Source: CAD feature listing. Evaluate the final solid. Frame: model axes, mm. Round coordinates to 2 decimals unless told otherwise and drop trailing zeros. Loops run counter-clockwise (first coordinate to the right, second up) from the corner with the lowest first, then second, coordinate; pieces in that order, holes last.
Item 1: Ray query, L1, parallel to Z at x = 5.45, y = 10; L2, parallel to Y at x = 4, z = 4; L3, parallel to Y at x = 1.8, z = -2. Return the intervals inside material, ascending.
Item 2: Section query B-B on z = 5. Return loops of the section in (x, y), then the cut area to 3 significant figures.
Item 3: Section query A-A on y = 10. Return loops of the section in (x, z), then the cut area to 3 significant figures.
Item 4: Section query D-D on y = 12.25. Return loops of the section in (x, z).
Item 5: Pull-direction query (Y, two-part tool) for faces 1 (the flat face through (3, 0, 12)), 2 (the cylindrical face through (2.96, 0.21, -0.43)), 3 (the flat face through (3, 0.2, 13)); classes: released by +Y, released by -Y, zero draft, split by the parting line, or undercut.
Item 6: Section query C-C on x = 5.5. Return loops of the section in (y, z).
Autodesk Inventor part; units mm, degrees
ref_plane "YZ Plane" through (0, 0, 0) normal (1, 0, 0) x (0, 1, 0)
ref_plane "XZ Plane" through (0, 0, 0) normal (0, 1, 0) x (-1, 0, 0)
ref_plane "XY Plane" through (0, 0, 0) normal (0, 0, 1) x (1, 0, 0)
sketch "Sketch1" plane through (0, 0, 0) normal (0, 0, 1) x (1, 0, 0)
  line L0 (0, 0) -> (6, 0)
  line L1 (6, 0) -> (6, 0.2)
  line L2 (6, 0.2) -> (0, 0.2)
  line L3 (0, 0.2) -> (0, 0)
  dimension "d0" = 0.2
  dimension "d1" = 6
extrude "Extrusion1" add sketch "Sketch1" along normal blind 10
sketch "Sketch2" plane through (0, 0, 0) normal (1, 0, 0) x (0, 1, 0)
  line L0 (0, 0) -> (0.2, 0)
  line L1 (0, 0) -> (10, 0)
  circle A0 centre (10, 0) radius 10
  circle A1 centre (10, 0) radius 9.8
  dimension "d4" = 10
extrude "Extrusion2" add sketch "Sketch2" along normal up to surface (6 mm away)
sketch "Sketch3" plane through (0, 0, 10) normal (0, 0, 1) x (1, 0, 0)
  line L0 (0, 0) -> (0, 0.2)
  line L1 (6, 0) -> (0, 0)
  line L2 (6, 0.2) -> (6, 0)
  line L3 (0, 0.2) -> (6, 0.2)
extrude "Extrusion3" add sketch "Sketch3" along normal blind 15
properties part number "FoilCoil2"
Data:
1. L1: z = -10 to -9.8, 9.8 to 10
1. L2: y = 0 to 0.2, 0.83 to 1.05, 18.95 to 19.17
1. L3: y = 0.2 to 0.41, 19.59 to 19.8
2. outline: (0, 0) - (6, 0) - (6, 0.2) - (0, 0.2) - close; (0, 1.34) - (6, 1.34) - (6, 1.57) - (0, 1.57) - close; (0, 18.43) - (6, 18.43) - (6, 18.66) - (0, 18.66) - close
2. area: 3.98 mm2
3. outline: (0, -10) - (6, -10) - (6, -9.8) - (0, -9.8) - close; (0, 9.8) - (6, 9.8) - (6, 10) - (0, 10) - close
3. area: 2.40 mm2
4. outline: (0, -9.74) - (6, -9.74) - (6, -9.54) - (0, -9.54) - close; (0, 9.54) - (6, 9.54) - (6, 9.74) - (0, 9.74) - close
5. face 1: released by -Y
5. face 2: undercut
5. face 3: undercut
6. outline: (0, 0) arc R10 ccw (long way) to (0.2, 1.99) - (0.2, 25) - (0, 25) - close; hole circle Ø19.6 at (10, 0)
